Design review of the part built by this model. Coordinates are the model's own, in mm. Round coordinates to 2 decimals unless told otherwise and drop trailing zeros. Order: outer loops, then holes, each group sorted by start corner. A loop starts at its lowest first (then second) coordinate and runs counter-clockwise, first axis right, second up. Notation, with made-up numbers: (3, 61.25) - (8, 61.25) arc R17 ccw to (8, 86.25) - close; hole circle Ø11 at (74.25, -40). An arc over 180 degrees is marked (long way). Answer as a JSON object with one key per item and string values. Group by question number.
from build123d import *

# Parameters (mm, degrees)
F0_W     = 279.4
F0_H     = 279.4
F1_DEPTH = 6.35
F2_R     = 1.905
F3_DEPTH = 5.08
F4_R     = 4.7625
F5_DEPTH = 6.351


with BuildPart() as f1:
    # F0 (on Top) → F1 (new body)
    with BuildSketch(Plane.XY):
        with Locations((139.7, 139.7)):
            Rectangle(F0_W, F0_H)
    extrude(amount=F1_DEPTH)

    # F2 (on face) → F3 (cut)
    with BuildSketch(Plane(origin=(0, 0, 0), x_dir=(1, 0, 0), z_dir=(0, 0, -1))):
        with Locations((38.1, -38.1)):
            Circle(F2_R)
        with Locations((88.9, -38.1)):
            Circle(F2_R)
        with Locations((139.7, -38.1)):
            Circle(F2_R)
        with Locations((241.3, -38.1)):
            Circle(F2_R)
        with Locations((190.5, -38.1)):
            Circle(F2_R)
        with Locations((38.1, -88.9)):
            Circle(F2_R)
        with Locations((88.9, -88.9)):
            Circle(F2_R)
        with Locations((139.7, -88.9)):
            Circle(F2_R)
        with Locations((190.5, -88.9)):
            Circle(F2_R)
        with Locations((241.3, -88.9)):
            Circle(F2_R)
        with Locations((38.1, -139.7)):
            Circle(F2_R)
        with Locations((88.9, -139.7)):
            Circle(F2_R)
        with Locations((139.7, -139.7)):
            Circle(F2_R)
        with Locations((190.5, -139.7)):
            Circle(F2_R)
        with Locations((241.3, -139.7)):
            Circle(F2_R)
        with Locations((241.3, -190.5)):
            Circle(F2_R)
        with Locations((190.5, -190.5)):
            Circle(F2_R)
        with Locations((139.7, -190.5)):
            Circle(F2_R)
        with Locations((88.9, -190.5)):
            Circle(F2_R)
        with Locations((38.1, -190.5)):
            Circle(F2_R)
        with Locations((38.1, -241.3)):
            Circle(F2_R)
        with Locations((88.9, -241.3)):
            Circle(F2_R)
        with Locations((139.7, -241.3)):
            Circle(F2_R)
        with Locations((190.5, -241.3)):
            Circle(F2_R)
        with Locations((241.3, -241.3)):
            Circle(F2_R)
    extrude(amount=-F3_DEPTH, mode=Mode.SUBTRACT)

    # F4 (on face) → F5 (cut, through all)
    with BuildSketch(Plane(origin=(0, 0, 0), x_dir=(1, 0, 0), z_dir=(0, 0, -1))):
        with Locations((19.05, -19.05)):
            Circle(F4_R)
        with Locations((260.35, -260.35)):
            Circle(F4_R)
        with Locations((19.05, -260.35)):
            Circle(F4_R)
        with Locations((260.35, -19.05)):
            Circle(F4_R)
    extrude(amount=-F5_DEPTH, mode=Mode.SUBTRACT)


solid = f1.part
1. To check wall thickness, follow line 1 (X direction, y = 38.1, z = 1.25) (3 decimals); line 2 (X direction, y = 260.5, z = 6.25). State the ranges of each line that lie inside material, in increasing order. Write a range as from..to.
2. Take a section at A-A, the plane x = 260.35. Give the boundary of the cut face in (y, z).
3. Clearance check with a flat-ended pin moving along its axis: P1, Ø1.9, axis at x = 139.5, y = 89.5, coming from the -Z side. State where the tip first meets the part, or that it passes through.
4. Mouldability with a two-part tool opening along X and no side actions: class faces 1 (the flat face through (0, 138, 3)), 2 (the flat face through (138, 279.4, 3)), 3 (the cylindrical face through (15.27, 263.25, 3.13)) as pulls with the +X half, pulls with the -X half, needs draft (parallel to the pull), parting line crosses it, or undercut.
Response values:
{
 "1": {"line 1": "0..36.195, 40.005..86.995, 90.805..137.795, 141.605..188.595, 192.405..239.395, 243.205..279.4", "line 2": "0..14.29, 23.81..255.59, 265.11..279.4"},
 "2": {"outline": "(0, 0) - (14.29, 0) - (14.29, 6.35) - (0, 6.35) - close; (23.81, 0) - (255.59, 0) - (255.59, 6.35) - (23.81, 6.35) - close; (265.11, 0) - (279.4, 0) - (279.4, 6.35) - (265.11, 6.35) - close"},
 "3": {"P1": "z = 5.08"},
 "4": {"face 1": "pulls with the -X half", "face 2": "needs draft", "face 3": "undercut"}
}
